Answer from the drawing. Dimensions are ordinates in mm from the lowest x, y and z of the part. A direction names the side the tool comes from. Give positions to 0.01 mm unless a question says otherwise; leave off trailing zeros. Loops run counter-clockwise (first coordinate to the right, second up) from the corner with the lowest first, then second, coordinate; pieces in that order, holes last. Notation, with made-up numbers: M 46.25,-5.5 L 93.25,-5.5 A25 cw 93.25,25.5 Z; hole C -24.5,-12.75 d6. An arc over 180 degrees is marked long. Use a Markdown table: item, result.
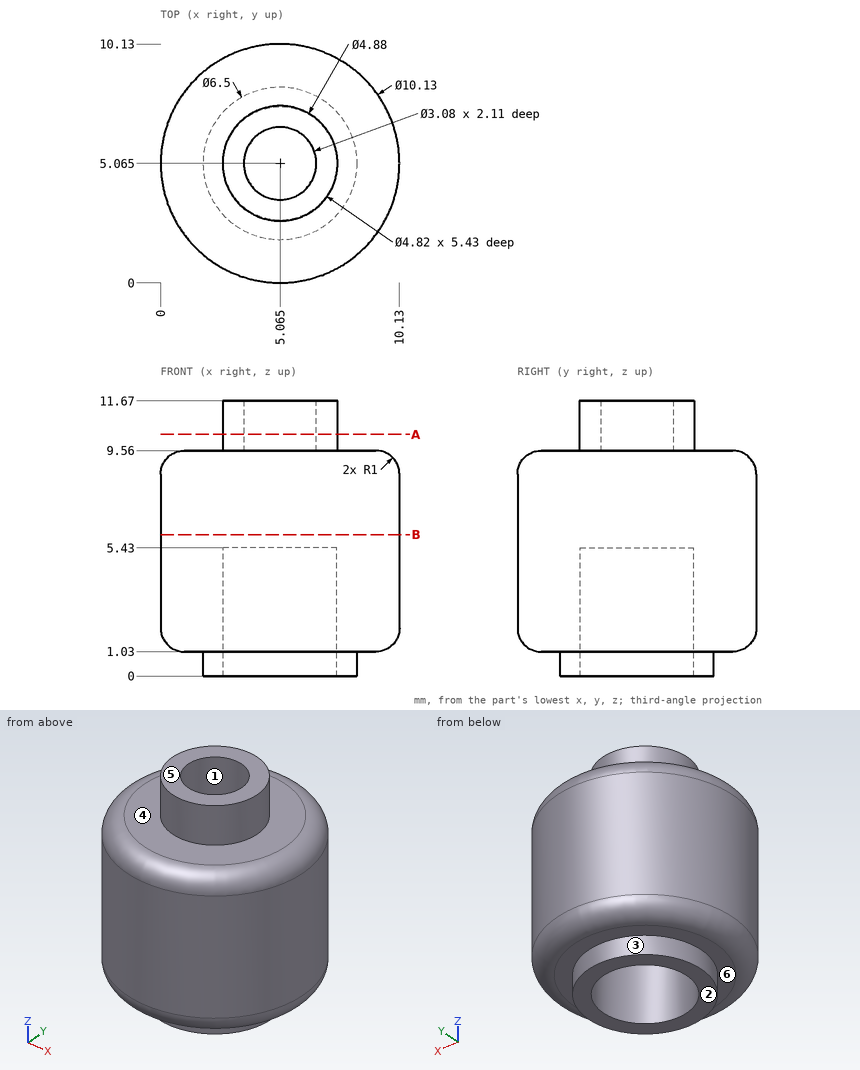
(1) The mould has two halves that part along X. Classify the marked faces 1, 2 and 3: released by +X, released by -X, zero draft, split by the parting line, or undercut.
Entries:
| item | result |
|---|---|
| face 1 | undercut |
| face 2 | zero draft |
| face 3 | split by the parting line |
(2) Which of the six approach directions +Z, -Z, +X, -X, +Y, -Y give full straight-line access (tool end or side, diameter ignored) to the marked faces 4, 5 and 6?
Entries:
| item | result |
|---|---|
| face 4 | +Z |
| face 5 | +Z, +X, -X, +Y, -Y |
| face 6 | -Z |
(3) A cutting plane is placed at B-B (z = 6). Write down the section's boundary in (x, y) (3 decimals), and give its area (3 significant figures).
Entries:
| item | result |
|---|---|
| outline | C 5.065,5.065 d10.13 |
| area | 80.6 mm² |
(4) Consider probe 1 along Z at (x, y) = (1.75, 2.75); probe 2 along Z at (x, y) = (6, 3.5); probe 3 along Y at (x, z) = (6.25, 1.25). Determine where each line is inside the solid, lowest interval first. Write a range as [from, to].
Entries:
| item | result |
|---|---|
| probe 1 | z = [1.03, 9.56] |
| probe 2 | z = [5.43, 11.67] |
| probe 3 | y = [0.53, 2.97], [7.16, 9.6] |
(5) Given P1, Ø3, axis at x = 3.5, z = 10.5, coming from the -Y side; P2, Ø3, axis at x = 5.065, y = 5.065, coming from the +Z side; P3, Ø1, axis at x = 8.5, y = 7, coming from the -Z side, each flat-ended and moving along its own axis, determine where each tip first touches the part or whether it passes through.
Entries:
| item | result |
|---|---|
| P1 | stops at y = 0.27 |
| P2 | stops at z = 9.56 |
| P3 | stops at z = 1.03 |
(6) A cutting plane is placed at A-A (z = 10.25). Write down the section's boundary in (x, y) (3 decimals), and give its area (3 significant figures).
Entries:
| item | result |
|---|---|
| outline | C 5.065,5.065 d4.88; hole C 5.065,5.065 d3.08 |
| area | 11.3 mm² |
